Source: three-view drawing plus pictorial views. Frame: mm from the lowest corner of the part. A direction names the side the tool comes from. Give positions to 0.01 mm unless a question says otherwise; leave off trailing zeros. Write each loop counter-clockwise with the first axis right and the second up, starting at its lowest first coordinate (ties: lowest second). Pieces come first, ordered by that corner, then holes. Notation, with made-up numbers: M 87.25,20 L 119.25,20 A28 ccw 119.25,49 Z; hole C -3.5,22 d3. An arc over 180 degrees is marked long. Return JSON: item names as keys, results as strings.
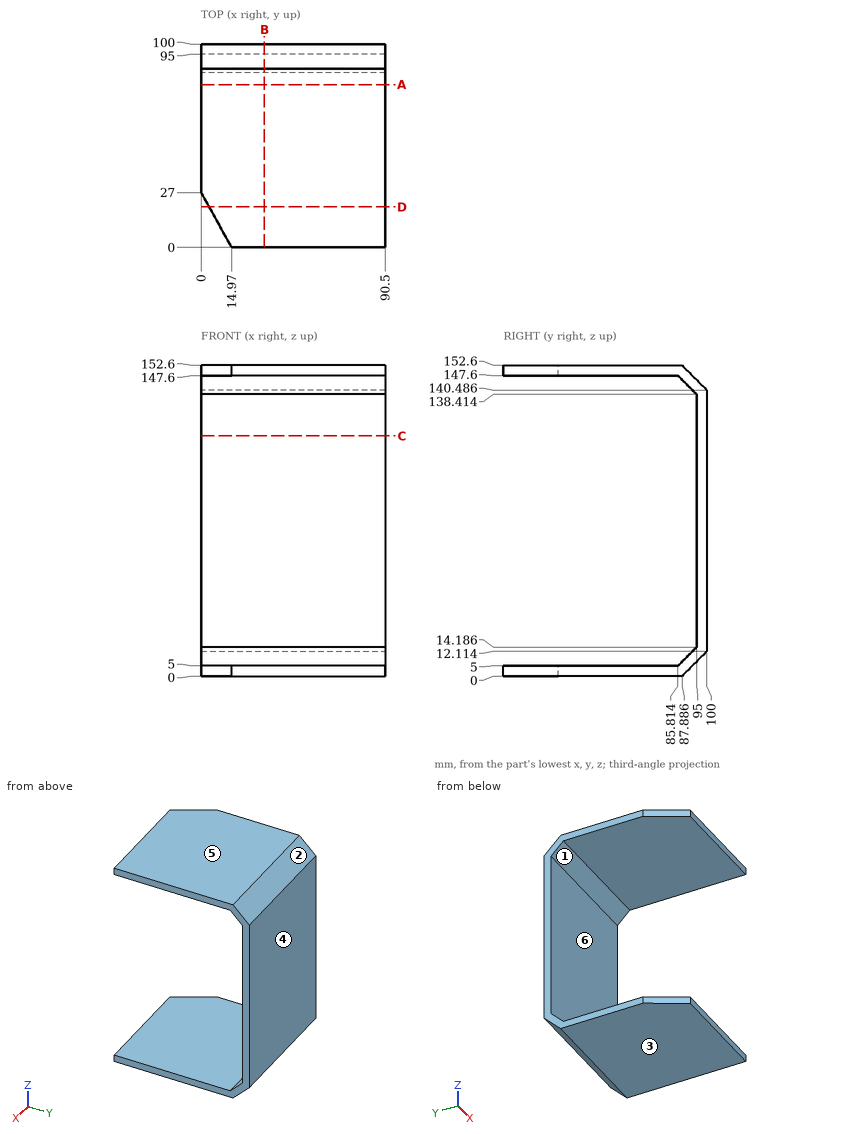
1) Cut plane C-C, the plane z = 118. Return the cut outline in (x, y).
Numbers:
{"outline": "M 0,95 L 90.5,95 L 90.5,100 L 0,100 Z"}
2) Line query: line 1 (Z direction, x = 26, y = 48); line 2 (Y direction, x = 81, z = 68); line 3 (Z direction, x = 22.5, y = 87.5) (1 decimal). Output: solid intervals per line, ascending. Write a range as [from, to].
Numbers:
{"line 1": "z = [0, 5], [147.6, 152.6]", "line 2": "y = [95, 100]", "line 3": "z = [0, 6.7], [145.9, 152.6]"}
3) Draft query along Z for the marked faces 3, 4, 5 and 6. Return one class per face: released by +Z, released by -Z, zero draft, split by the parting line, or undercut.
Numbers:
{"face 3": "released by -Z", "face 4": "zero draft", "face 5": "released by +Z", "face 6": "undercut"}
4) Set-up query: the marked faces 1 and 2. Return all of +Z, -Z, +X, -X, +Y, -Y with unobstructed straight access to the full face (end or side cutting, diameter ignored); none if empty.
Numbers:
{"face 1": "+X, -X, -Y", "face 2": "+Z, +X, -X, +Y"}
5) Cut plane D-D, the plane y = 20. Return the cut outline in (x, z).
Numbers:
{"outline": "M 3.88,0 L 90.5,0 L 90.5,5 L 3.88,5 Z; M 3.88,147.6 L 90.5,147.6 L 90.5,152.6 L 3.88,152.6 Z"}
6) Cut plane B-B, the plane x = 31. Return the cut outline in (y, z) (1 decimal), then the cut area to 3 significant figures.
Numbers:
{"outline": "M 0,0 L 87.9,0 L 100,12.1 L 100,140.5 L 87.9,152.6 L 0,152.6 L 0,147.6 L 85.8,147.6 L 95,138.4 L 95,14.2 L 85.8,5 L 0,5 Z", "area": "1,650 mm²"}
7) Cut plane A-A, the plane y = 80. Return the cut outline in (x, z), then the cut area to 3 significant figures.
Numbers:
{"outline": "M 0,0 L 90.5,0 L 90.5,5 L 0,5 Z; M 0,147.6 L 90.5,147.6 L 90.5,152.6 L 0,152.6 Z", "area": "905 mm²"}
8) Contact query for a flat-ended pin moving along its axis: pin 1 Ø4 at (x, y) = (78.5, 40.5) entering from -Z. Output: stop coordinate, or through.
Numbers:
{"pin 1": "stops at z = 0"}
